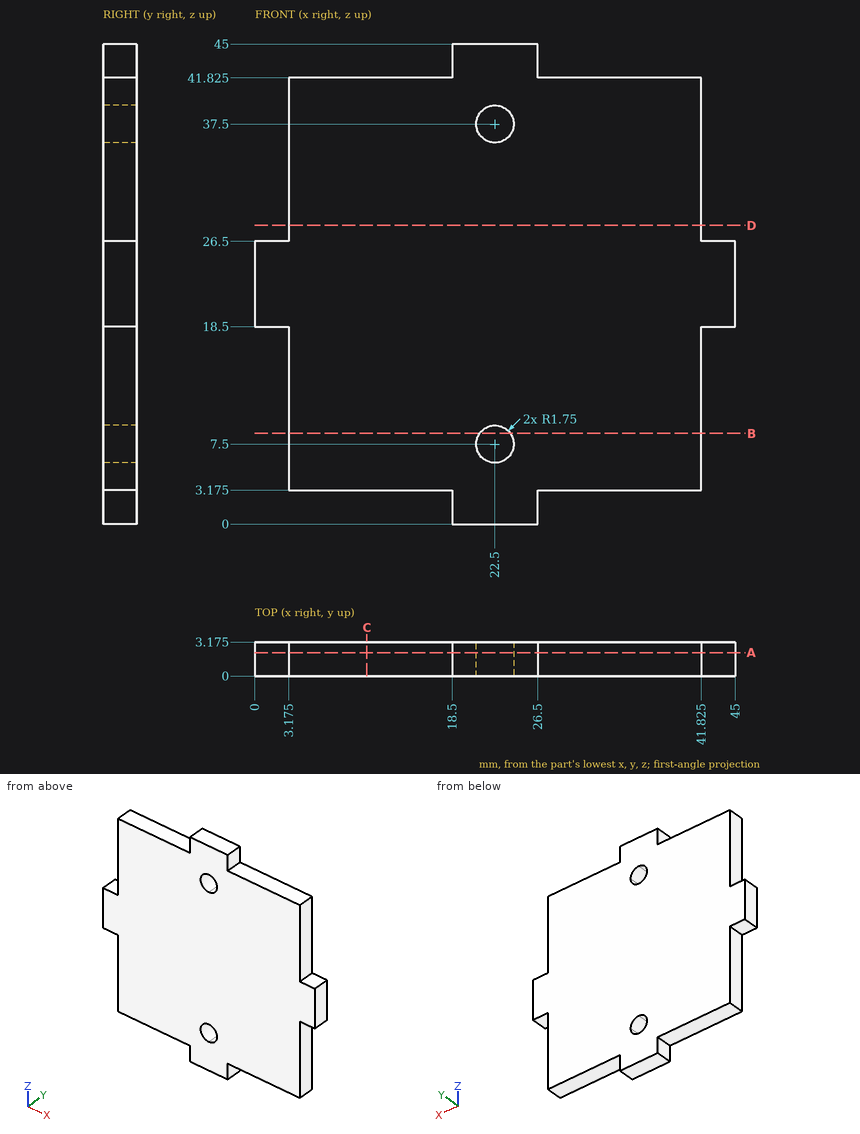
Drawing for the job (mm, zero at the part's lowest x, y, z). Give positions to 0.01 mm unless a question says otherwise; leave off trailing zeros. Order: outer loops, then holes, each group sorted by start corner. A loop starts at its lowest first (then second) coordinate and runs counter-clockwise, first axis right, second up. Notation, with made-up numbers: M 10,14 L 35,14 A20 cw 35,33 Z; hole C 26,53.25 d10. An arc over 180 degrees is marked long. Put each result on its own line as item: value. Start each with the question number.
(1) Drill centre lines: line 1 along Z through (x, y) = (23.5, 2.95); line 2 along X through (y, z) = (0.75, 37.5) (3 decimals); line 3 along Z through (x, y) = (35, 2.9) (3 decimals). Where is each one in solid material? Low to high.
(2) Flat gauge pins, fed straight in: pin 1 Ø1 at (x, y) = (1.5, 1.5) entering from +Z; pin 2 Ø1.6 at (x, y) = (9, 1.5) entering from +Z (3 decimals); pin 3 Ø1 at (y, z) = (1.5, 10) entering from -X (3 decimals). Where does each tip first touch, or does it go through?
(3) Saw through at D-D, the plane z = 28. Write the cut outline in (x, y) (3 decimals).
(4) Saw through at A-A, the plane y = 2.2. Write the cut outline in (x, z) (3 decimals).
(5) Saw through at C-C, the plane x = 10.5. Write the cut outline in (y, z) (3 decimals).
(6) Saw through at B-B, the plane z = 8.5. Write the cut outline in (x, y) (3 decimals), then the cut area to 3 significant figures.
Check result:
1. line 1: z = 0 to 6.06, 8.94 to 36.06, 38.94 to 45
1. line 2: x = 3.175 to 20.75, 24.25 to 41.825
1. line 3: z = 3.175 to 41.825
2. pin 1: stops at z = 26.5
2. pin 2: stops at z = 41.825
2. pin 3: stops at x = 3.175
3. outline: M 3.175,0 L 41.825,0 L 41.825,3.175 L 3.175,3.175 Z
4. outline: M 0,18.5 L 3.175,18.5 L 3.175,3.175 L 18.5,3.175 L 18.5,0 L 26.5,0 L 26.5,3.175 L 41.825,3.175 L 41.825,18.5 L 45,18.5 L 45,26.5 L 41.825,26.5 L 41.825,41.825 L 26.5,41.825 L 26.5,45 L 18.5,45 L 18.5,41.825 L 3.175,41.825 L 3.175,26.5 L 0,26.5 Z; hole C 22.5,7.5 d3.5; hole C 22.5,37.5 d3.5
5. outline: M 0,3.175 L 3.175,3.175 L 3.175,41.825 L 0,41.825 Z
6. outline: M 3.175,0 L 21.064,0 L 21.064,3.175 L 3.175,3.175 Z; M 23.936,0 L 41.825,0 L 41.825,3.175 L 23.936,3.175 Z
6. area: 114 mm2
